Read the model definition and answer for the solid it produces. Units are mm, in the model's axes. A direction names the side the tool comes from. Coordinates: 2 decimals unless noted, no trailing zeros. Order: outer loops, then holes, each group sorted by start corner. A loop starts at its lowest first (then second) coordinate and runs counter-clockwise, first axis right, second up. Notation, with made-up numbers: (52, 81) - (81, 81) arc R23 ccw to (81, 109) - close; hole circle Ø6 at (20.25, 32.5). An arc over 180 degrees is marked (long way). Use one line per item in the form item = value. Start each with the question number.
from build123d import *

# Parameters (mm, degrees)
SKETCH_W        = 9.5
SKETCH_H        = 9.5
PAD_DEPTH       = 11
SKETCH001_R     = 4.075
PAD001_DEPTH    = 14.07
SKETCH005_R     = 5.75
POCKET002_DEPTH = 2.3
SKETCH006_R     = 5.15
POCKET003_DEPTH = 4.8
SKETCH007_R     = 2.5
POCKET_DEPTH    = 1
SKETCH008_R     = 0.75
POCKET004_DEPTH = 5
CHAMFER_SIZE    = 0.5
SKETCH009_R     = 3.85
PAD002_DEPTH    = 2
SKETCH010_R     = 2.28
PAD003_DEPTH    = 1
SKETCH011_W     = 2.06
SKETCH011_H     = 0.5
PAD004_DEPTH    = 6


with BuildPart() as part:
    # Sketch → Pad (new body)
    with BuildSketch(Plane.XY):
        Rectangle(SKETCH_W, SKETCH_H)
    extrude(amount=-PAD_DEPTH)

    # Sketch001 (on Face5 of Pad) → Pad001 (join)
    with BuildSketch(Plane.XY):
        Circle(SKETCH001_R)
    extrude(amount=PAD001_DEPTH)

    # Sketch005 → Pocket002 (cut)
    with BuildSketch(Plane(origin=(0, 0, -11), x_dir=(1, 0, 0), z_dir=(0, 0, -1))):
        Circle(SKETCH005_R)
    extrude(amount=-POCKET002_DEPTH, mode=Mode.SUBTRACT)

    # Sketch006 (on Face6 of Pocket002) → Pocket003 (cut)
    with BuildSketch(Plane(origin=(0, 0, -8.7), x_dir=(1, 0, 0), z_dir=(0, 0, -1))):
        Circle(SKETCH006_R)
    extrude(amount=-POCKET003_DEPTH, mode=Mode.SUBTRACT)

    # Sketch007 (on Face24 of Pocket003) → Pocket (cut)
    with BuildSketch(Plane.XY.offset(14.07)):
        Circle(SKETCH007_R)
    extrude(amount=-POCKET_DEPTH, mode=Mode.SUBTRACT)

    # Sketch008 (on Face26 of Pocket) → Pocket004 (cut)
    with BuildSketch(Plane.XY.offset(13.07)):
        Circle(SKETCH008_R)
    extrude(amount=-POCKET004_DEPTH, mode=Mode.SUBTRACT)

    # Chamfer
    chamfer_edges = [part.edges().sort_by_distance(p)[0] for p in [
        (-0.75, 0, 13.07),
    ]]
    chamfer(chamfer_edges, length=CHAMFER_SIZE)

    # Sketch009 (on Face17 of Chamfer) → Pad002 (join)
    with BuildSketch(Plane(origin=(0, 0, -3.9), x_dir=(1, 0, 0), z_dir=(0, 0, -1))):
        Circle(SKETCH009_R)
    extrude(amount=PAD002_DEPTH)

    # Sketch010 (on Face31 of Pad002) → Pad003 (join)
    with BuildSketch(Plane(origin=(0, 0, -5.9), x_dir=(1, 0, 0), z_dir=(0, 0, -1))):
        Circle(SKETCH010_R)
    extrude(amount=PAD003_DEPTH)

    # Sketch011 (on Face33 of Pad003) → Pad004 (join)
    with BuildSketch(Plane(origin=(0, 0, -6.9), x_dir=(1, 0, 0), z_dir=(0, 0, -1))):
        Rectangle(SKETCH011_W, SKETCH011_H)
    extrude(amount=PAD004_DEPTH)


solid = part.part
Q1. A cutting plane is placed at A-A (z = -4.75). Give the vertices of the cut face in (x, y), then the cut area to 3 significant figures.
Q2. Consider probe 1 along Y at (x, z) = (0, 9.25) (3 decimals); probe 2 along Y at (x, z) = (0, 13.75) (3 decimals); probe 3 along Z at (x, y) = (3.25, 1). Determine where each line is inside the solid, lowest interval first.
Q3. Given P1, Ø2.5, axis at x = 1, y = -0.5, coming from the +Z side; P2, Ø0.8, axis at x = 2.5, y = -4, coming from the -Z side; P3, Ø1.6, axis at x = 0, y = 0, coming from the +Z side, each flat-ended and moving along its own axis, determine where each tip first touches the part or whether it passes through.
Q4. Which of the six approach directions +Z, -Z, +X, -X, +Y, -Y give full straight-line access (tool end or side, diameter ignored) to faces 4 (the cylindrical face through (-0.75, 0.03, 10.35)), 5 (the cylindrical face through (3.661, -3.622, -6.334)), 6 (the flat face through (2, 2, 14.07)), 7 (the flat face through (0, -0.25, -10))?
Q5. A cutting plane is placed at D-D (z = 6.25). Give the vertices of the cut face in (x, y) (3 decimals).
Q6. For a pull along Y with two mould halves and no side action, classify faces 1 (the flat face through (4.75, 0, -3)), 2 (the cylindrical face through (-0.83, 3.76, -4.89)), 3 (the flat face through (0, -4.75, -3)) as +Y half, -Y half, draft (parallel to the pull), parting line (faces both ways), or undercut.
Result sheet:
q1.outline = (-4.75, -4.75) - (-1.99, -4.75) arc R5.15 cw to (-4.75, -1.99) - close; (-4.75, 1.99) arc R5.15 cw to (-1.99, 4.75) - (-4.75, 4.75) - close; circle Ø7.7 at (0, 0); (1.99, -4.75) - (4.75, -4.75) - (4.75, -1.99) arc R5.15 cw to start; (1.99, 4.75) arc R5.15 cw to (4.75, 1.99) - (4.75, 4.75) - close
q1.area = 57.8 mm^2
q2.probe_1 = -4.075 to -0.75, 0.75 to 4.075
q2.probe_2 = -4.075 to -2.5, 2.5 to 4.075
q2.probe_3 = -5.9 to 14.07
q3.P1 = 13.07
q3.P2 = -3.9
q3.P3 = 12.62
q4.face_4 = +Z
q4.face_5 = -Z
q4.face_6 = +Z, +X, -X, +Y, -Y
q4.face_7 = -Z, +X, -X, -Y
q5.outline = circle Ø8.15 at (0, 0)
q6.face_1 = draft
q6.face_2 = undercut
q6.face_3 = -Y half
